Check sheet for the modelled part. Datum: model origin and axes. Units: mm. Round coordinates to 2 decimals unless told otherwise and drop trailing zeros. Loops run counter-clockwise (first coordinate to the right, second up) from the corner with the lowest first, then second, coordinate; pieces in that order, holes last. Notation, with made-up numbers: M 84,-2.75 L 112,-2.75 A15 cw 112,25.25 Z; hole C -5,-12.75 d2. An arc over 180 degrees is marked long. Write item = value, one per line. Start each with the question number.
(1) Scan lines: L1, parallel to X at y = -2.4, z = 20; L2, parallel to Z at x = 96, y = -1.45; L3, parallel to X at y = -3.6, z = 26.5. Record each from-to range of solid material in increasing order. Write a range as from..to.
(2) Cross-section at B-B on x = 96. Record the boundary of the cut face in (y, z).
(3) Cross-section at A-A on y = -0.8. Record the boundary of the cut face in (x, z), plus the area to 3 significant figures.
(4) Go/stop test with a flat-tipped pin: P1, Ø7, axis at x = 116, z = 20, coming from the +Y side. Record where the tip stops, or that it passes through.
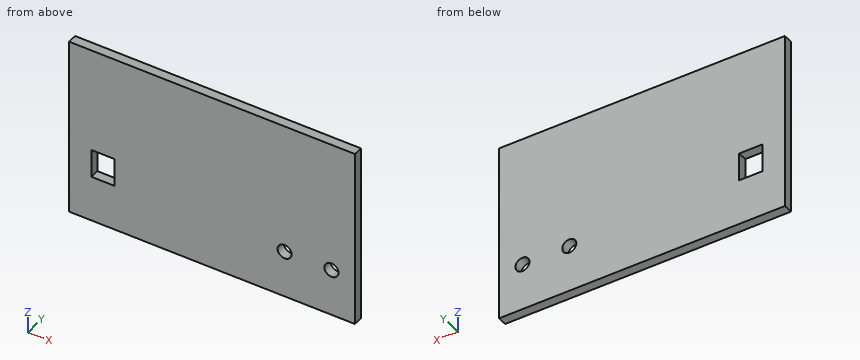
from build123d import *

# Parameters (mm, degrees)
SKETCH002_W   = 122
SKETCH002_H   = 76
PAD001_DEPTH  = 4
SKETCH003_W   = 10
SKETCH003_H   = 12
POCKET_DEPTH  = 4.001
SKETCH008_R   = 3
HOLE002_DEPTH = 4.001


with BuildPart() as part:
    # Sketch002 → Pad001 (new body)
    with BuildSketch(Plane.XZ):
        with Locations((65, 38)):
            Rectangle(SKETCH002_W, SKETCH002_H)
    extrude(amount=PAD001_DEPTH)

    # Sketch003 (on Face6 of Pad001) → Pocket (cut, through all)
    with BuildSketch(Plane.XZ.offset(4)):
        with Locations((18.5, 25.5)):
            Rectangle(SKETCH003_W, SKETCH003_H)
    extrude(amount=-POCKET_DEPTH, mode=Mode.SUBTRACT)

    # Sketch008 (on Face4 of Pocket) → Hole002 (cut, through all)
    with BuildSketch(Plane(origin=(0, 0, 0), x_dir=(1, 0, 0), z_dir=(0, 1, 0))):
        with Locations((116, -20)):
            Circle(SKETCH008_R)
        with Locations((96, -20)):
            Circle(SKETCH008_R)
    extrude(amount=-HOLE002_DEPTH, mode=Mode.SUBTRACT)


solid = part.part
Result:
q1.L1 = 4..13.5, 23.5..93, 99..113, 119..126
q1.L2 = 0..17, 23..76
q1.L3 = 4..13.5, 23.5..126
q2.outline = M -4,0 L 0,0 L 0,17 L -4,17 Z; M -4,23 L 0,23 L 0,76 L -4,76 Z
q3.outline = M 4,0 L 126,0 L 126,76 L 4,76 Z; hole M 13.5,19.5 L 23.5,19.5 L 23.5,31.5 L 13.5,31.5 Z; hole C 96,20 d6; hole C 116,20 d6
q3.area = 9,100 mm^2
q4.P1 = 0
